Here's how the part is built. I have some questions about the finished solid (model axes, mm). Coordinates: 2 decimals unless noted, no trailing zeros. Order: outer loops, then holes, each group sorted by start corner. A loop starts at its lowest first (then second) coordinate and runs counter-clockwise, first axis right, second up. Notation, with made-up numbers: (75.5, 8.25) - (99.5, 8.25) arc R25 ccw to (99.5, 35.25) - close; hole circle Ø1 at (55, 4.5). An arc over 180 degrees is marked (long way). Answer in a Markdown table with one row per item. Add a question column.
Item 1: I want a section at B-B (z = 4.75). Please give me the cut outline in (x, y), plus the area to 3 significant figures.
Item 2: I want a section at C-C (y = 125.5). Please give me the cut outline in (x, z), plus the area to 3 significant figures.
Item 3: Will these pins go through, and if not, where does the flat tip stop? pin 1 Ø8 at (y, z) = (-7.5, -3) entering from +X; pin 2 Ø3 at (x, y) = (43, -30.5) entering from -Z; pin 3 Ø8 at (y, z) = (-2, -6.5) entering from -X; pin 4 Ø4 at (x, z) = (-45.5, -3.5) entering from -Y.
Item 4: I want a section at A-A (x = 43). Please give me the cut outline in (y, z).
Item 5: If I drill on line 1 along Y through (x, z) = (13.5, 4.5); line 2 along Z through (x, y) = (62.5, -86.5); line 3 along Y through (x, z) = (0, -7.5), over which ranges is the centre line in solid material (lowest first)? Write a range as from..to.
```python
from build123d import *

# Parameters (mm, degrees)
F0_W     = 135
F0_H     = 300
F1_DEPTH = 8
F3_DEPTH = 50
F5_D     = 12
F5_DEPTH = 5
F5_TIP   = 3.6051637142
F7_DEPTH = 25


with BuildPart() as f1:
    # F0 (on Top) → F1 (new body)
    with BuildSketch(Plane.XY):
        Rectangle(F0_W, F0_H)
    extrude(amount=F1_DEPTH)

    # F2 (on Right) → F3 (join, symmetric)
    with BuildSketch(Plane.YZ):
        Polygon((0, -10), (0, 0), (-7.9979246179, 0), (-15, -10), align=None)
        Polygon((7.9979246179, 0), (0, 0), (0, -10), (15, -10), align=None)
    extrude(amount=F3_DEPTH, both=True)

    # F5
    with Locations(Plane(origin=(0, 0, -10), x_dir=(1, 0, 0), z_dir=(0, 0, -1))):
        with Locations((0, 0)):
            Hole(F5_D / 2, depth=F5_DEPTH)
            with Locations((0, 0, -(F5_DEPTH + F5_TIP / 2))):  # 118° drill point
                Cone(0, F5_D / 2, F5_TIP, mode=Mode.SUBTRACT)

    # F6 (on face) → F7 (cut)
    with BuildSketch(Plane.XY.offset(8)):
        with BuildLine():
            ThreePointArc((59, -135), (57.8284271247, -132.1715728753), (55, -131))
            Line((55, -131), (55, -139))
            ThreePointArc((55, -139), (57.8284271247, -137.8284271247), (59, -135))
        make_face()
        with BuildLine():
            Line((55, -139), (55, -131))
            ThreePointArc((55, -131), (51, -135), (55, -139))
        make_face()
        with BuildLine():
            Line((55, -131), (-55, -131))
            ThreePointArc((-55, -131), (-52.1715728753, -132.1715728753), (-51, -135))
            ThreePointArc((-51, -135), (-52.1715728753, -137.8284271247), (-55, -139))
            Line((-55, -139), (55, -139))
            ThreePointArc((55, -139), (51, -135), (55, -131))
        make_face()
        with BuildLine():
            ThreePointArc((-51, -135), (-52.1715728753, -132.1715728753), (-55, -131))
            Line((-55, -131), (-55, -139))
            ThreePointArc((-55, -139), (-52.1715728753, -137.8284271247), (-51, -135))
        make_face()
        with BuildLine():
            Line((-55, -139), (-55, -131))
            ThreePointArc((-55, -131), (-59, -135), (-55, -139))
        make_face()
        with BuildLine():
            Line((55, 139), (55, 131))
            ThreePointArc((55, 131), (57.8284271247, 132.1715728753), (59, 135))
            ThreePointArc((59, 135), (57.8284271247, 137.8284271247), (55, 139))
        make_face()
        with BuildLine():
            ThreePointArc((55, 139), (51, 135), (55, 131))
            Line((55, 131), (55, 139))
        make_face()
        with BuildLine():
            ThreePointArc((-51, 135), (-52.1715728753, 132.1715728753), (-55, 131))
            Line((-55, 131), (55, 131))
            ThreePointArc((55, 131), (51, 135), (55, 139))
            Line((55, 139), (-55, 139))
            ThreePointArc((-55, 139), (-52.1715728753, 137.8284271247), (-51, 135))
        make_face()
        with BuildLine():
            ThreePointArc((-55, 139), (-59, 135), (-55, 131))
            Line((-55, 131), (-55, 139))
        make_face()
        with BuildLine():
            Line((-55, 139), (-55, 131))
            ThreePointArc((-55, 131), (-52.1715728753, 132.1715728753), (-51, 135))
            ThreePointArc((-51, 135), (-52.1715728753, 137.8284271247), (-55, 139))
        make_face()
    extrude(amount=-F7_DEPTH, mode=Mode.SUBTRACT)


solid = f1.part
```
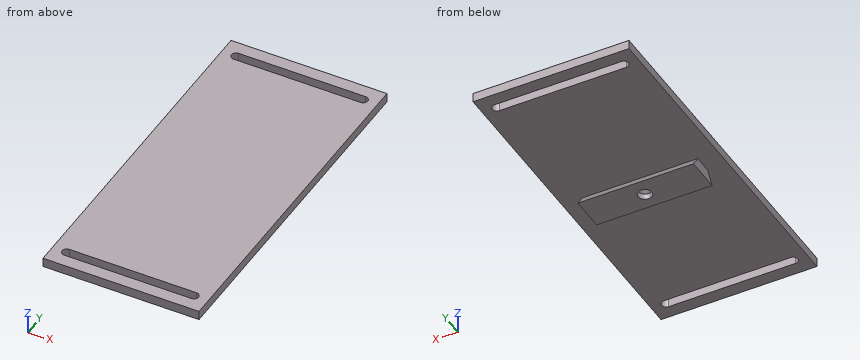
Values follow:
| question | item | result |
|---|---|---|
| 1 | outline | (-67.5, -150) - (67.5, -150) - (67.5, 150) - (-67.5, 150) - close; hole (-55, -139) - (55, -139) arc R4 ccw to (55, -131) - (-55, -131) arc R4 ccw to start; hole (-55, 131) - (55, 131) arc R4 ccw to (55, 139) - (-55, 139) arc R4 ccw to start |
| 1 | area | 38,600 mm^2 |
| 2 | outline | (-67.5, 0) - (67.5, 0) - (67.5, 8) - (-67.5, 8) - close |
| 2 | area | 1,080 mm^2 |
| 3 | pin 1 | stops at x = 67.5 |
| 3 | pin 2 | stops at z = 0 |
| 3 | pin 3 | stops at x = -50 |
| 3 | pin 4 | stops at y = -11.85 |
| 4 | outline | (-150, 0) - (-139, 0) - (-139, 8) - (-150, 8) - close; (-131, 0) - (-8, 0) - (-15, -10) - (15, -10) - (8, 0) - (131, 0) - (131, 8) - (-131, 8) - close; (139, 0) - (150, 0) - (150, 8) - (139, 8) - close |
| 5 | line 1 | y = -150..-139, -131..131, 139..150 |
| 5 | line 2 | z = 0..8 |
| 5 | line 3 | y = -13.25..-6, 6..13.25 |
